Check sheet for the modelled part. Datum: model origin and axes. Units: mm. Face numbers are marked on the shaded views. A direction names the side the tool comes from. Give positions to 0.01 mm unless a question says otherwise; leave off trailing zeros. Write each loop counter-clockwise with the first axis right and the second up, starting at its lowest first coordinate (ties: lowest second). Pieces come first, ordered by that corner, then holes. Notation, with made-up numbers: (75.25, 21) - (115.25, 21) arc R32 ccw to (115.25, 54) - close; hole circle Ø11 at (66.5, 84). An arc over 180 degrees is marked (long way). Return JSON: item names as keys, results as strings. Group by question number.
```python
from build123d import *

# Parameters (mm, degrees)
SKETCH1_W           = 20
SKETCH1_H           = 12
BOSS_EXTRUDE1_DEPTH = 30
SKETCH2_W           = 40
SKETCH2_H           = 40
BOSS_EXTRUDE2_DEPTH = 20
FILLET1_R           = 10


with BuildPart() as part:
    # Sketch1 → Boss-Extrude1 (new body)
    with BuildSketch(Plane.XY):
        with Locations((-20, -6)):
            Rectangle(SKETCH1_W, SKETCH1_H)
    extrude(amount=BOSS_EXTRUDE1_DEPTH)

    # Sketch2 → Boss-Extrude2 (add)
    with BuildSketch(Plane.XY):
        with Locations((-10, 8)):
            Rectangle(SKETCH2_W, SKETCH2_H)
    extrude(amount=-BOSS_EXTRUDE2_DEPTH)

    # Fillet1
    fillet1_edges = [part.edges().sort_by_distance(p)[0] for p in [
        (10, 28, -10),
        (-20, 0, 30),
        (-20, 0, 0),
    ]]
    fillet(fillet1_edges, radius=FILLET1_R)


solid = part.part
```
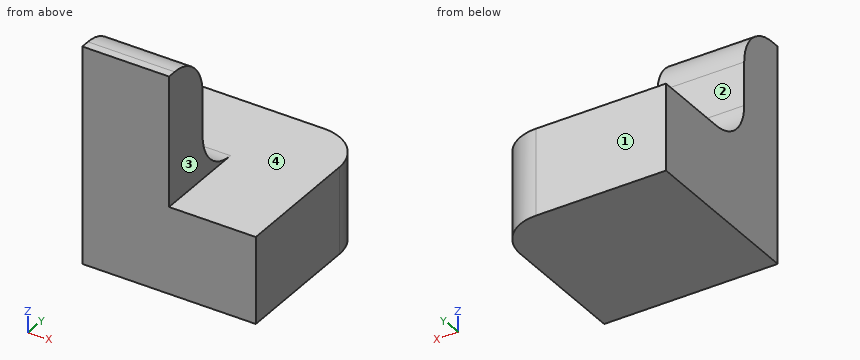
Item 1: Section check C-C on z = 18. Record the cut outline in (x, y).
Item 2: Access from +Z, -Z, +X, -X, +Y, -Y to the whole of each face (thin tool, end or side, straight path). Record for the marked faces 1, 2, 3 and 4.
Item 3: Material ranges on line 1 along Z through (x, y) = (2.5, 20.5); line 2 along X through (y, z) = (-8, 12); line 3 along Z through (x, y) = (-21.5, 2.5), recorded low to high. Write a range as from..to.
Item 4: Depth check by flat-ended pin: pin 1 (3 mm diameter, centred on x = -22.5, z = 14, fed in from +Y); pin 2 (6.5 mm diameter, centred on y = 0, z = 11, fed in from +X); pin 3 (5 mm diameter, centred on x = 4, y = 0.5, fed in from +Z). Enter the tip coordinate at first touch or a pass-through.
Item 5: Section check A-A on x = -23.5. Record the cut outline in (y, z).
Item 6: Section check D-D on y = 24. Record the cut outline in (x, z), plus the area to 3 significant figures.
Item 7: Section check B-B on y = -4. Record the cut outline in (x, z).
Reply:
{
 "1": {"outline": "(-30, -12) - (-10, -12) - (-10, 0) - (-30, 0) - close"},
 "2": {"face 1": "+Z, -Z, +X, -X, +Y", "face 2": "+Z, +X, -X, +Y", "face 3": "+Z, +X, +Y, -Y", "face 4": "+Z, +X, +Y"},
 "3": {"line 1": "-20..0", "line 2": "-30..-10", "line 3": "-20..3.39"},
 "4": {"pin 1": "y = 0", "pin 2": "x = -10", "pin 3": "z = 0"},
 "5": {"outline": "(-12, -20) - (28, -20) - (28, 0) - (10, 0) arc R10 cw to (0, 10) - (0, 20) arc R10 ccw to (-10, 30) - (-12, 30) - close"},
 "6": {"outline": "(-30, -20) - (8, -20) - (8, 0) - (-30, 0) - close", "area": "760 mm²"},
 "7": {"outline": "(-30, -20) - (10, -20) - (10, 0) - (-10, 0) - (-10, 28) - (-30, 28) - close"}
}
